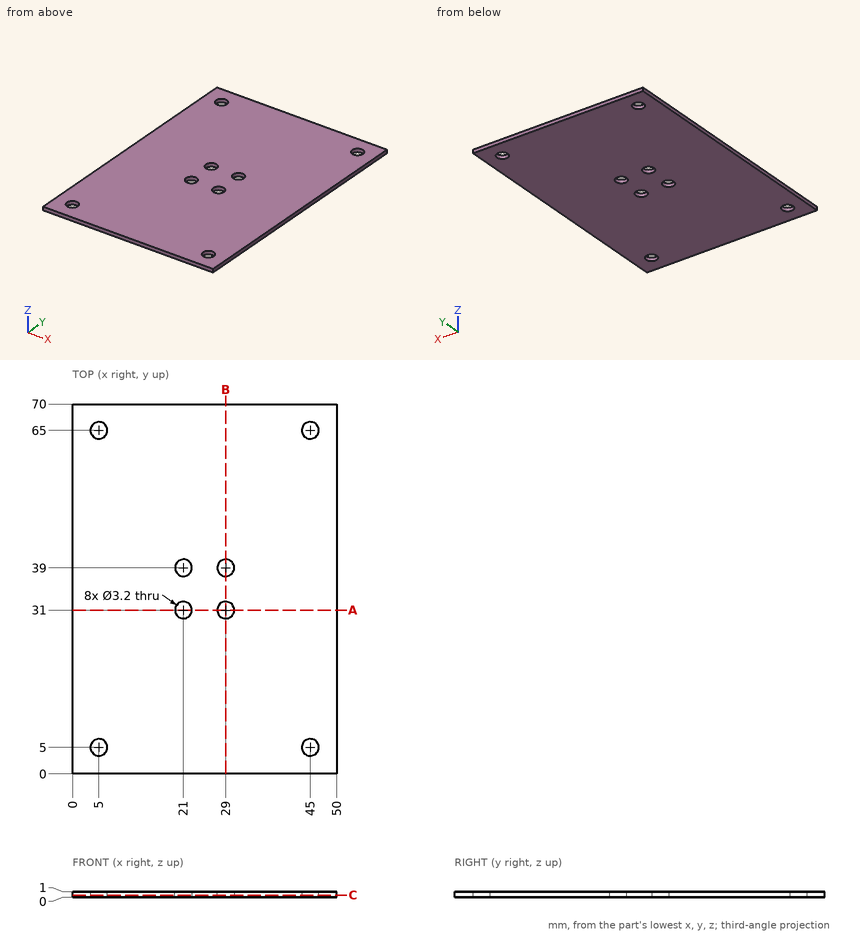
Study the drawing (mm; zero at the part's minimum x, y, z) and answer. Coordinates: 2 decimals unless noted, no trailing zeros. Write each loop counter-clockwise with the first axis right and the second up, starting at its lowest first coordinate (ties: lowest second). Pieces come first, ordered by that corner, then holes.
Q1. Section C-C, the plane z = 0.4 is taken. Give the number of separate pieces and of enclosed holes in the cut face, then the cut area to 3 significant figures.
Returned:
separate pieces: 1
enclosed holes: 8
area: 3,440 mm2
Q2. Find the intervals of material crossed by line 1 along Y through (x, z) = (29, 0.6); line 2 along Y through (x, z) = (45, 0.6); line 3 along X through (y, z) = (40, 0.15), in increasing order.
Returned:
line 1: y = 0 to 29.4, 32.6 to 37.4, 40.6 to 70
line 2: y = 0 to 3.4, 6.6 to 63.4, 66.6 to 70
line 3: x = 0 to 19.75, 22.25 to 27.75, 30.25 to 50
Q3. Section A-A, the plane y = 31 is taken. Write down the section's boundary in (x, z).
Returned:
outline: (0, 0) - (19.4, 0) - (19.4, 1) - (0, 1) - close; (22.6, 0) - (27.4, 0) - (27.4, 1) - (22.6, 1) - close; (30.6, 0) - (50, 0) - (50, 1) - (30.6, 1) - close
Q4. Section B-B, the plane x = 29 is taken. Write down the section's boundary in (y, z), then the cut area to 3 significant figures.
Returned:
outline: (0, 0) - (29.4, 0) - (29.4, 1) - (0, 1) - close; (32.6, 0) - (37.4, 0) - (37.4, 1) - (32.6, 1) - close; (40.6, 0) - (70, 0) - (70, 1) - (40.6, 1) - close
area: 63.6 mm2
